Input: part model. Units: mm. Frame: model coordinates. Give positions to 0.01 mm unless a question says otherwise; leave off trailing zeros.
from build123d import *

# Parameters (mm, degrees)
SKETCH_1_W            = 500
SKETCH_1_H            = 220
EXTRUDE_1_DEPTH       = 50
CUT_EXTRUDE_1_DEPTH   = 65
SKETCH_3_W            = 24.993501938
SKETCH_3_H            = 24.754329671
EXTRUDE_2_DEPTH       = 50
SKETCH_4_W            = 557.488309353
SKETCH_4_H            = 263.064748201
SKETCH_4_W_2          = 497.488309353
SKETCH_4_H_2          = 203.064748201
CUT_EXTRUDE_1_2_DEPTH = 84
SCALE_1_SCALE         = 1.5
SKETCH_8_W            = 822.232464029
SKETCH_8_H            = 353.597122302
SKETCH_8_W_2          = 722.232464029
SKETCH_8_H_2          = 253.597122302
CUT_EXTRUDE_2_DEPTH   = 180
SKETCH_9_W            = 725
SKETCH_9_H            = 254
SKETCH_9_W_2          = 708.249145706
SKETCH_9_H_2          = 240.894932361
EXTRUDE_4_DEPTH       = 75


with BuildPart() as part:
    # Эскиз1 → Бобышка-Вытянуть1 (new body)
    with BuildSketch(Plane.XY):
        with Locations((315.178539616, -203.237931197)):
            Rectangle(SKETCH_1_W, SKETCH_1_H)
        Polygon((203.546220768, -131.339893042), (185.513397027, -144.433418222), (140.884350264, -144.433418222), (131.736418609, -131.339893042), align=None, mode=Mode.SUBTRACT)
        Polygon((159.677066091, -260.404641243), (87.867263933, -260.404641243), (105.900087674, -247.311116064), (150.529134437, -247.311116064), align=None, mode=Mode.SUBTRACT)
        Polygon((116.392443789, -207.416781531), (103.766544509, -244.593040524), (85.938307098, -258.534137646), (104.994062494, -202.419029733), (111.160879041, -198.678022538), align=None, mode=Mode.SUBTRACT)
        Polygon((109.933361055, -187.922626855), (128.287677602, -133.911835488), (136.67571717, -147.706799517), (124.225177602, -184.41543261), (113.060609257, -193.066511747), align=None, mode=Mode.SUBTRACT)
        Polygon((181.158630839, -203.997267143), (162.86276753, -257.832698797), (154.445501343, -244.066961387), (166.92526753, -207.299875056), (178.20674235, -198.678022538), align=None, mode=Mode.SUBTRACT)
        Polygon((174.874907818, -183.947806711), (187.354674005, -147.239173618), (205.124458178, -133.444209589), (186.770141631, -187.455000956), (180.106472566, -193.066511747), align=None, mode=Mode.SUBTRACT)
        Polygon((172.098379041, -189.325504553), (176.833091271, -195.872267143), (167.626706379, -202.419029733), (119.695051703, -202.419029733), (114.931112854, -195.872267143), (124.166724365, -189.325504553), align=None, mode=Mode.SUBTRACT)
        Polygon((188.173019329, -260.404641243), (192.615465372, -247.311116064), (205.708990552, -247.311116064), (201.266544509, -260.404641243), align=None, mode=Mode.SUBTRACT)
        Polygon((220.585339473, -165.00895779), (225.057012134, -151.91543261), (238.150537314, -151.91543261), (233.678864652, -165.00895779), align=None, mode=Mode.SUBTRACT)
        Polygon((347.574997746, -131.339893042), (329.542174005, -144.433418222), (284.913127242, -144.433418222), (275.765195588, -131.339893042), align=None, mode=Mode.SUBTRACT)
        Polygon((303.70584307, -260.404641243), (231.896040911, -260.404641243), (249.928864652, -247.311116064), (294.557911415, -247.311116064), align=None, mode=Mode.SUBTRACT)
        Polygon((260.421220768, -207.416781531), (247.795321487, -244.593040524), (229.967084077, -258.534137646), (249.022839473, -202.419029733), (255.189656019, -198.678022538), align=None, mode=Mode.SUBTRACT)
        Polygon((253.962138034, -187.922626855), (272.31645458, -133.911835488), (280.704494149, -147.706799517), (268.25395458, -184.41543261), (257.089386235, -193.066511747), align=None, mode=Mode.SUBTRACT)
        Polygon((325.187407818, -203.997267143), (306.891544509, -257.832698797), (298.474278321, -244.066961387), (310.954044509, -207.299875056), (322.235519329, -198.678022538), align=None, mode=Mode.SUBTRACT)
        Polygon((318.903684796, -183.947806711), (331.383450983, -147.239173618), (349.153235156, -133.444209589), (330.798918609, -187.455000956), (324.135249545, -193.066511747), align=None, mode=Mode.SUBTRACT)
        Polygon((316.127156019, -189.325504553), (320.86186825, -195.872267143), (311.655483357, -202.419029733), (263.723828681, -202.419029733), (258.959889832, -195.872267143), (268.195501343, -189.325504553), align=None, mode=Mode.SUBTRACT)
        Polygon((446.711688393, -131.339893042), (428.678864652, -144.433418222), (384.04981789, -144.433418222), (374.901886235, -131.339893042), align=None, mode=Mode.SUBTRACT)
        Polygon((402.842533717, -260.404641243), (331.032731559, -260.404641243), (349.0655553, -247.311116064), (393.694602063, -247.311116064), align=None, mode=Mode.SUBTRACT)
        Polygon((359.557911415, -207.416781531), (346.932012134, -244.593040524), (329.103774724, -258.534137646), (348.15953012, -202.419029733), (354.326346667, -198.678022538), align=None, mode=Mode.SUBTRACT)
        Polygon((353.098828681, -187.922626855), (371.453145228, -133.911835488), (379.841184796, -147.706799517), (367.390645228, -184.41543261), (356.226076883, -193.066511747), align=None, mode=Mode.SUBTRACT)
        Polygon((424.324098465, -203.997267143), (406.028235156, -257.832698797), (397.610968969, -244.066961387), (410.090735156, -207.299875056), (421.372209976, -198.678022538), align=None, mode=Mode.SUBTRACT)
        Polygon((418.040375444, -183.947806711), (430.520141631, -147.239173618), (448.289925804, -133.444209589), (429.935609257, -187.455000956), (423.271940192, -193.066511747), align=None, mode=Mode.SUBTRACT)
        Polygon((415.263846667, -189.325504553), (419.998558897, -195.872267143), (410.792174005, -202.419029733), (362.860519329, -202.419029733), (358.09658048, -195.872267143), (367.332191991, -189.325504553), align=None, mode=Mode.SUBTRACT)
        Polygon((545.848379041, -131.339893042), (527.8155553, -144.433418222), (483.186508537, -144.433418222), (474.038576883, -131.339893042), align=None, mode=Mode.SUBTRACT)
        Polygon((501.979224365, -260.404641243), (430.169422206, -260.404641243), (448.202245947, -247.311116064), (492.83129271, -247.311116064), align=None, mode=Mode.SUBTRACT)
        Polygon((458.694602063, -207.416781531), (446.068702782, -244.593040524), (428.240465372, -258.534137646), (447.296220768, -202.419029733), (453.463037314, -198.678022538), align=None, mode=Mode.SUBTRACT)
        Polygon((452.235519329, -187.922626855), (470.589835875, -133.911835488), (478.977875444, -147.706799517), (466.527335875, -184.41543261), (455.36276753, -193.066511747), align=None, mode=Mode.SUBTRACT)
        Polygon((523.460789113, -203.997267143), (505.164925804, -257.832698797), (496.747659616, -244.066961387), (509.227425804, -207.299875056), (520.508900624, -198.678022538), align=None, mode=Mode.SUBTRACT)
        Polygon((517.177066091, -183.947806711), (529.656832278, -147.239173618), (547.426616451, -133.444209589), (529.072299904, -187.455000956), (522.408630839, -193.066511747), align=None, mode=Mode.SUBTRACT)
        Polygon((514.400537314, -189.325504553), (519.135249545, -195.872267143), (509.928864652, -202.419029733), (461.997209976, -202.419029733), (457.233271127, -195.872267143), (466.468882638, -189.325504553), align=None, mode=Mode.SUBTRACT)
    extrude(amount=EXTRUDE_1_DEPTH)

    # Эскиз2 → Cut-Extrude 1 (cut)
    with BuildSketch(Plane.XY.offset(50)):
        Polygon((225.057012134, -151.91543261), (238.150537314, -151.91543261), (233.678864652, -165.00895779), (220.585339473, -165.00895779), align=None)
        Polygon((199.643902872, -226.731116064), (212.737428052, -226.731116064), (208.26575539, -239.824641243), (195.17223021, -239.824641243), align=None)
    extrude(amount=-CUT_EXTRUDE_1_DEPTH, mode=Mode.SUBTRACT)

    # Эскиз3 → Бобышка-Вытянуть2 (add)
    with BuildSketch(Plane.XY.offset(50)):
        with Locations((196.457377331, -256.289777907)):
            Rectangle(SKETCH_3_W, SKETCH_3_H)
    extrude(amount=-EXTRUDE_2_DEPTH)

    # Эскиз4 → Cut-Extrude 1 2 (cut)
    with BuildSketch(Plane.XY.offset(50)):
        with Locations((316.682461775, -195.872267142)):
            Rectangle(SKETCH_4_W, SKETCH_4_H)
        with Locations((316.682461775, -195.872267142)):
            Rectangle(SKETCH_4_W_2, SKETCH_4_H_2, mode=Mode.SUBTRACT)
    extrude(amount=-CUT_EXTRUDE_1_2_DEPTH, mode=Mode.SUBTRACT)


with BuildPart() as part_1:
    # Масштаб1: scaled about (314.289349403, -195.861916492, 25)
    add(part.part.scale(SCALE_1_SCALE).moved(Location((-157.144674702, 97.930958246, -12.5))))

    # Эскиз8 → Вырез-Вытянуть-Тонкостенный2 (cut)
    with BuildSketch(Plane.XY.offset(62.5)):
        with Locations((317.879017961, -195.877442468)):
            Rectangle(SKETCH_8_W, SKETCH_8_H)
        with Locations((317.879017961, -195.877442468)):
            Rectangle(SKETCH_8_W_2, SKETCH_8_H_2, mode=Mode.SUBTRACT)
    extrude(amount=-CUT_EXTRUDE_2_DEPTH, mode=Mode.SUBTRACT)

    # Эскиз9 → Бобышка-Вытянуть4 (add)
    with BuildSketch(Plane.XY.offset(62.5)):
        with Locations((317.877785946, -195.878881317)):
            Rectangle(SKETCH_9_W, SKETCH_9_H)
        with Locations((317.250065853, -196.40613993)):
            Rectangle(SKETCH_9_W_2, SKETCH_9_H_2, mode=Mode.SUBTRACT)
    extrude(amount=-EXTRUDE_4_DEPTH)


solid = part_1.part
(1) Pin query (flat end, axial travel): pin 1 Ø5 at (x, y) = (309, -100.5) entering from -Z. Return the tip coordinate at first contact, or that it passes through.
Values follow:
pin 1: stops at z = -12.5
(2) Ray query, probe 1 along Y at (x, z) = (276, 22.5); probe 2 along X at (y, z) = (-195, -6.5); probe 3 along X at (y, z) = (-101, -4.5). Return the intervals inside material, ascending.
Values follow:
probe 1: y = -322.88 to -292.68, -273.04 to -205.7, -186.06 to -118.72, -99.08 to -68.88
probe 2: x = -44.62 to 16.49, 107.47 to 232.53, 323.51 to 381.24, 472.22 to 529.94, 620.92 to 680.38
probe 3: x = -44.62 to 41.8, 145.53 to 257.85, 361.57 to 406.55, 510.28 to 555.26, 658.98 to 680.38
(3) Cut plane A-A (z = 32.5). Count the separate pieces of the cut face and the enclosed holes in it, and give its area (3 significant figures).
Values follow:
separate pieces: 1
enclosed holes: 30
area: 140,000 mm2
